Can you work these out from the model? Positions are in its coordinate system, mm. Face numbers are marked on the shaded views. A direction names the side the tool comes from. Round coordinates to 2 decimals unless told otherwise and drop trailing zeros. Loops run counter-clockwise (first coordinate to the right, second up) from the corner with the lowest first, then second, coordinate; pieces in that order, holes last. Notation, with made-up numbers: M 35,2.5 L 55,2.5 A6 ccw 55,12.5 Z; hole C 19.25,17 d5. An arc over 180 degrees is marked long. Answer as CSV lines item,"result".
from build123d import *

# Parameters (mm, degrees)
SKETCH1_W           = 15
SKETCH1_H           = 10
SKETCH1_H_2         = 15
SKETCH1_W_2         = 10
BOSS_EXTRUDE1_DEPTH = 16.7
SKETCH2_R           = 6.5
CUT_EXTRUDE1_DEPTH  = 8.3
SKETCH3_R           = 6.5
CUT_EXTRUDE2_DEPTH  = 8.3
SKETCH4_R           = 6.5
CUT_EXTRUDE3_DEPTH  = 14.7
FILLET8_R           = 2
SKETCH5_W           = 42
SKETCH5_H           = 42
SKETCH5_R           = 2
SKETCH5_R_2         = 7.906463766
BOSS_EXTRUDE3_DEPTH = 5
FILLET9_R           = 1


with BuildPart() as part:
    # Sketch1 → Boss-Extrude1 (new body)
    with BuildSketch(Plane(origin=(0, 0, 0), x_dir=(1, 0, 0), z_dir=(0, 1, 0))):
        Rectangle(SKETCH1_W, SKETCH1_H)
        with Locations((0, 12.5)):
            Rectangle(SKETCH1_W, SKETCH1_H_2)
        with Locations((12.5, 12.5)):
            Rectangle(SKETCH1_W_2, SKETCH1_H_2)
    extrude(amount=BOSS_EXTRUDE1_DEPTH)

    # Sketch2 → Cut-Extrude1 (cut)
    with BuildSketch(Plane.XY.offset(5)):
        with Locations((0, 8.35)):
            Circle(SKETCH2_R)
    extrude(amount=-CUT_EXTRUDE1_DEPTH, mode=Mode.SUBTRACT)

    # Sketch3 → Cut-Extrude2 (cut)
    with BuildSketch(Plane(origin=(17.5, 0, 0), x_dir=(0, 0, -1), z_dir=(1, 0, 0))):
        with Locations((12.5, 8.35)):
            Circle(SKETCH3_R)
    extrude(amount=-CUT_EXTRUDE2_DEPTH, mode=Mode.SUBTRACT)

    # Sketch4 → Cut-Extrude3 (cut)
    with BuildSketch(Plane.XZ):
        with Locations(Location((0, -12.5, 0), (0, 0, 270))):
            Circle(SKETCH4_R)
    extrude(amount=-CUT_EXTRUDE3_DEPTH, mode=Mode.SUBTRACT)

    # Fillet8
    # the kernel refuses this fillet: 2 mm, written as the material it adds along each edge
    with BuildSketch(Plane(origin=(7.5, 0, -5), x_dir=(0, 0, 1), z_dir=(0, 1, 0))) as fillet8_piece_1:
        with BuildLine():
            CenterArc((FILLET8_R, FILLET8_R), FILLET8_R, 180, 90)
            Line((0, FILLET8_R), (0, 0))
            Line((0, 0), (FILLET8_R, 0))
        make_face()
    extrude(amount=16.7)
    # the kernel refuses this fillet: 2 mm, written as the material it takes off along each edge
    with BuildSketch(Plane(origin=(-5.5, 2, -18), x_dir=(0, 0, -1), z_dir=(-1, 0, 0))) as fillet8_2_piece_1_section:
        Polygon((0, 0), (FILLET8_R, 0), (FILLET8_R, FILLET8_R), (0, FILLET8_R), align=None)
    fillet8_2_piece_1 = extrude(amount=FILLET8_R, mode=Mode.PRIVATE)
    fillet8_2_piece_1 = fillet8_2_piece_1 - Plane(origin=(-5.5, 2, -18), x_dir=(0, 0.7071067811865475, 0.7071067811865475), z_dir=(-1, 0, 0)) * Sphere(FILLET8_R, mode=Mode.PRIVATE)
    add(fillet8_2_piece_1, mode=Mode.SUBTRACT)
    with BuildSketch(Plane(origin=(-5.5, 14.7, -18), x_dir=(0, 1, 0), z_dir=(-1, 0, 0))) as fillet8_2_piece_2_section:
        Polygon((0, 0), (FILLET8_R, 0), (FILLET8_R, FILLET8_R), (0, FILLET8_R), align=None)
    fillet8_2_piece_2 = extrude(amount=FILLET8_R, mode=Mode.PRIVATE)
    fillet8_2_piece_2 = fillet8_2_piece_2 - Plane(origin=(-5.5, 14.7, -18), x_dir=(0, -0.7071067811865475, 0.7071067811865475), z_dir=(-1, 0, 0)) * Sphere(FILLET8_R, mode=Mode.PRIVATE)
    add(fillet8_2_piece_2, mode=Mode.SUBTRACT)
    with BuildSketch(Plane(origin=(-7.5, 0, -18), x_dir=(0, 1, 0), z_dir=(0, 0, 1)), Plane(origin=(22.5, 16.7, -20), x_dir=(0, 0, 1), z_dir=(-1, 0, 0)), Plane(origin=(-7.5, 16.7, 10), x_dir=(0, -1, 0), z_dir=(0, 0, -1)), Plane(origin=(22.5, 0, -20), x_dir=(0, 1, 0), z_dir=(-1, 0, 0))) as fillet8_2_piece_3:
        with BuildLine():
            CenterArc((FILLET8_R, -FILLET8_R), FILLET8_R, 90, 90)
            Line((0, -FILLET8_R), (0, 0))
            Line((0, 0), (FILLET8_R, 0))
        make_face()
    extrude(amount=28, mode=Mode.SUBTRACT)
    with BuildSketch(Plane(origin=(-7.5, 2, -20), x_dir=(0, 0, 1), z_dir=(0, 1, 0))) as fillet8_2_piece_4:
        with BuildLine():
            CenterArc((FILLET8_R, FILLET8_R), FILLET8_R, 180, 90)
            Line((0, FILLET8_R), (0, 0))
            Line((0, 0), (FILLET8_R, 0))
        make_face()
    extrude(amount=12.7, mode=Mode.SUBTRACT)
    # the kernel refuses this fillet: 2 mm, written as the material it takes off along each edge
    with BuildSketch(Plane(origin=(9.5, 0, -5), x_dir=(0, 0, -1), z_dir=(1, 0, 0))) as fillet8_3_piece_1:
        with BuildLine():
            CenterArc((FILLET8_R, FILLET8_R), FILLET8_R, 180, 90)
            Line((0, FILLET8_R), (0, 0))
            Line((0, 0), (FILLET8_R, 0))
        make_face()
    extrude(amount=13, mode=Mode.SUBTRACT)
    with BuildSketch(Plane(origin=(7.5, 0, -3), x_dir=(-1, 0, 0), z_dir=(0, 0, 1))) as fillet8_3_piece_2:
        with BuildLine():
            CenterArc((FILLET8_R, -FILLET8_R), FILLET8_R, 90, 90)
            Line((0, -FILLET8_R), (0, 0))
            Line((0, 0), (FILLET8_R, 0))
        make_face()
    extrude(amount=13, mode=Mode.SUBTRACT)
    with BuildSketch(Plane(origin=(9.5, 0, -3), x_dir=(-1, 0, 0), z_dir=(0, 0, 1))) as fillet8_3_piece_3:
        with BuildLine():
            CenterArc((2 + FILLET8_R, -FILLET8_R), FILLET8_R, 90, 90)
            Line((2, -FILLET8_R), (2, 0))
            Line((2, 0), (2 + FILLET8_R, 0))
        make_face()
    revolve(axis=Axis((9.5, 0, -3), (0, -1, 0)), revolution_arc=90, mode=Mode.SUBTRACT)

    # Sketch5 → Boss-Extrude3 (add)
    with BuildSketch(Plane(origin=(0, 16.7, 0), x_dir=(1, 0, 0), z_dir=(0, 1, 0))):
        with Locations((28.5, -16)):
            Rectangle(SKETCH5_W, SKETCH5_H)
        with Locations(Location((12.5, 0, 0), (0, 0, 270))):
            Circle(SKETCH5_R, mode=Mode.SUBTRACT)
        with Locations(Location((12.5, -32, 0), (0, 0, 270))):
            Circle(SKETCH5_R, mode=Mode.SUBTRACT)
        with Locations(Location((44.5, -32, 0), (0, 0, 270))):
            Circle(SKETCH5_R, mode=Mode.SUBTRACT)
        with Locations(Location((44.5, 0, 0), (0, 0, 270))):
            Circle(SKETCH5_R, mode=Mode.SUBTRACT)
        with Locations(Location((28.5, -16, 0), (0, 0, 270))):
            Circle(SKETCH5_R_2, mode=Mode.SUBTRACT)
    extrude(amount=-BOSS_EXTRUDE3_DEPTH)

    # Fillet9
    fillet9_edges = [part.edges().sort_by_distance(p)[0] for p in [
        (17.5, 14.2, -5),
        (7.5, 14.2, 5),
        (49.5, 14.2, 37),
        (7.5, 14.2, 37),
        (49.5, 14.2, -5),
    ]]
    fillet(fillet9_edges, radius=FILLET9_R)


solid = part.part
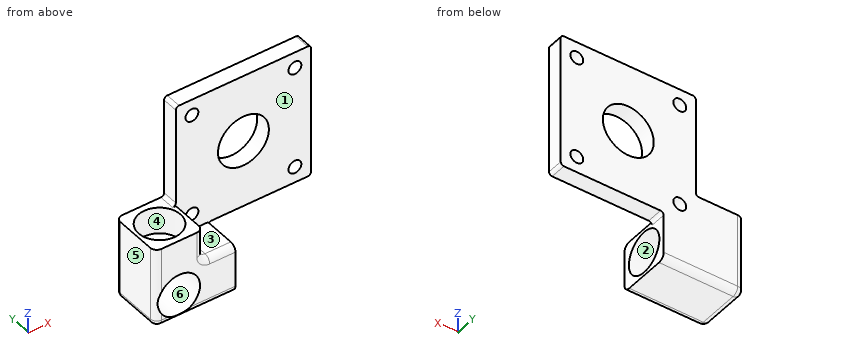
Item 1: If we section it at D-D on x = 44.5: Write out the boundary of the cut face in (y, z).
Output:
outline,"M 11.7,-5 L 16.7,-5 L 16.7,-2 L 11.7,-2 Z; M 11.7,2 L 16.7,2 L 16.7,30 L 11.7,30 Z; M 11.7,34 L 16.7,34 L 16.7,37 L 11.7,37 Z"
Item 2: On a 3-axis mill with a long thin cutter (end or side, diameter ignored), from which of +Z, -Z, +X, -X, +Y, -Y can I reach the whole of each face in a straight line? I mean the marked faces 4, 5 and 6. Say none if no direction works.
Output:
face 4,"+Z"
face 5,"+Z, -Z, -X, +Y, -Y"
face 6,"-Y"
Item 3: If we section it at C-C on x = 28.5: Write out the boundary of the cut face in (y, z), then the cut area to 3 significant figures.
Output:
outline,"M 11.7,-5 L 16.7,-5 L 16.7,8.09 L 11.7,8.09 Z; M 11.7,23.91 L 16.7,23.91 L 16.7,37 L 11.7,37 Z"
area,"131 mm2"
Item 4: If we section it at B-B on y = 6.75: Write out the boundary of the cut face in (x, z).
Output:
outline,"M -7.5,-18 A2 ccw -5.5,-20 L 17.5,-20 L 17.5,-18.8 L 9.2,-18.8 L 9.2,-6.2 L 17.5,-6.2 L 17.5,-5 L 9.5,-5 A2 cw 7.5,-3 L 7.5,5 L 6.3,5 L 6.3,-3.3 L -6.3,-3.3 L -6.3,5 L -7.5,5 Z; hole C 0,-12.5 d13"
Item 5: If I drill on line 1 along X through (y, z) = (15.45, 16); line 2 along X through (y, z) = (7, -10); line 3 along X through (y, z) = (13.7, 0), over which ranges is the centre line in solid material (lowest first)? Write a range as from..to.
Output:
line 1,"x = 7.5..20.59, 36.41..49.5"
line 2,"x = -7.5..-6, 6..9.2"
line 3,"x = -7.5..-3.69, 3.69..10.5, 14.5..42.5, 46.5..49.5"
Item 6: If we section it at A-A on z = 0: Write out the boundary of the cut face in (x, y).
Output:
outline,"M -7.5,2 A2 ccw -5.5,0 L 5.5,0 A2 ccw 7.5,2 L 7.5,11.7 L 10.5,11.7 L 10.5,16.7 L -5.5,16.7 A2 ccw -7.5,14.7 Z; M 14.5,11.7 L 42.5,11.7 L 42.5,16.7 L 14.5,16.7 Z; M 46.5,11.7 L 49.5,11.7 L 49.5,16.7 L 46.5,16.7 Z; hole C 0,8.35 d13"
Item 7: Will these pins go through, and if not, where does the flat tip stop? pin 1 (5 mm diameter, centred on y = 5.5, z = -1.5, fed in from +X); pin 2 (10 mm diameter, centred on x = 20.5, y = 3, fed in from +Z); pin 3 (4 mm diameter, centred on x = 37, y = 13.5, fed in from -Z).
Output:
pin 1,"stops at x = 7.77"
pin 2,"stops at z = -5"
pin 3,"stops at z = -5"
Item 8: We'd pull the mould along Z, two halves only. Please class the marked faces 1, 2 and 3: released by +Z, released by -Z, zero draft, split by the parting line, or undercut.
Output:
face 1,"zero draft"
face 2,"undercut"
face 3,"released by +Z"
